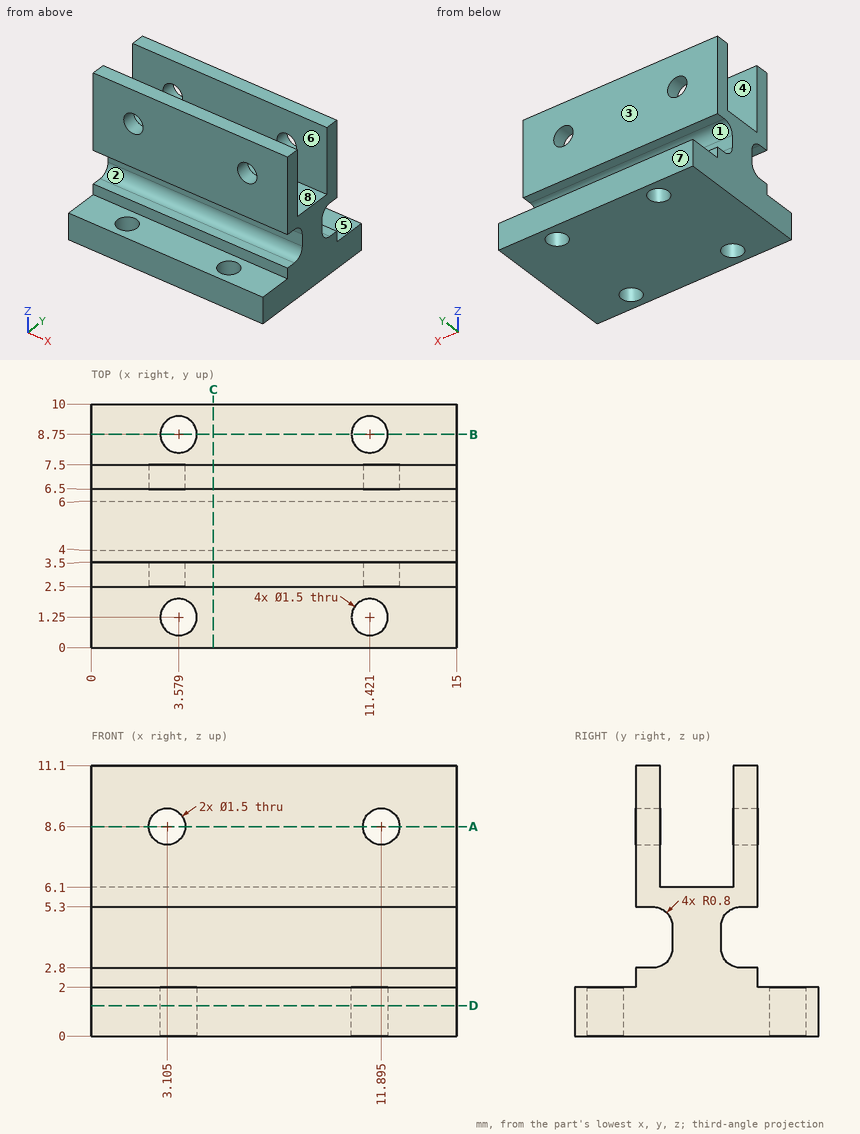
Job drawing, mm, ordinate dimensions from the low corner. One solid piece. A direction names the side the tool comes from. Round coordinates to 2 decimals unless told otherwise and drop trailing zeros. Loops run counter-clockwise (first coordinate to the right, second up) from the corner with the lowest first, then second, coordinate; pieces in that order, holes last. Notation, with made-up numbers: (86.25, 88) -> (99.25, 88) arc R30 cw to (99.25, 111) -> close; hole circle Ø7 at (51, 87). An arc over 180 degrees is marked (long way). Use a Markdown table: item, result.
1) Cut at A-A, the plane z = 8.6. List the corners of the cut face in (x, y) (1 decimal).
The answers:
| item | result |
|---|---|
| outline | (0, 2.5) -> (2.4, 2.5) -> (2.4, 3.5) -> (0, 3.5) -> close; (0, 6.5) -> (2.4, 6.5) -> (2.4, 7.5) -> (0, 7.5) -> close; (3.9, 2.5) -> (11.1, 2.5) -> (11.1, 3.5) -> (3.9, 3.5) -> close; (3.9, 6.5) -> (11.1, 6.5) -> (11.1, 7.5) -> (3.9, 7.5) -> close; (12.6, 2.5) -> (15, 2.5) -> (15, 3.5) -> (12.6, 3.5) -> close; (12.6, 6.5) -> (15, 6.5) -> (15, 7.5) -> (12.6, 7.5) -> close |
2) Pull direction Y, two halves, no side cores. Call the marked faces 5, 6, 7 and 8: pulls with the +Y half, pulls with the -Y half, needs draft (parallel to the pull), parting line crosses it, or undercut.
The answers:
| item | result |
|---|---|
| face 5 | needs draft |
| face 6 | undercut |
| face 7 | pulls with the +Y half |
| face 8 | undercut |
3) Tool access for the marked faces 1, 2, 3 and 4: list every direction of +Z, -Z, +X, -X, +Y, -Y with a clear straight run to the whole face (end or side of a thin tool).
The answers:
| item | result |
|---|---|
| face 1 | +X, -X, +Y |
| face 2 | +X, -X, -Y |
| face 3 | +Z, +X, -X, +Y |
| face 4 | +Z, +X, -X |
4) Cut at D-D, the plane z = 1.25. List the corners of the cut face in (x, y).
The answers:
| item | result |
|---|---|
| outline | (0, 0) -> (15, 0) -> (15, 10) -> (0, 10) -> close; hole circle Ø1.5 at (3.58, 1.25); hole circle Ø1.5 at (3.58, 8.75); hole circle Ø1.5 at (11.42, 1.25); hole circle Ø1.5 at (11.42, 8.75) |
5) Drop flat-ended pins along their axis: pin 1 Ø5.5 at (x, z) = (10, 7.5) entering from -Y; pin 2 Ø1.7 at (x, z) = (11.9, 8.6) entering from +Y; pin 3 Ø1 at (x, z) = (9, 4) entering from -Y; pin 4 Ø1.7 at (x, y) = (3.58, 8.75) entering from -Z. Give the stop position or say it passes through.
The answers:
| item | result |
|---|---|
| pin 1 | stops at y = 2.5 |
| pin 2 | stops at y = 7.5 |
| pin 3 | stops at y = 3.99 |
| pin 4 | stops at z = 0 |
6) Probe line 1 (Y direction, x = 9.75, z = 6.75); line 2 (Z direction, x = 3.5, y = 2.75); line 3 (X direction, y = 9, z = 1) (1 decimal). List the from-to ranges inside material, lowest first. Write a range as [from, to].
The answers:
| item | result |
|---|---|
| line 1 | y = [2.5, 3.5], [6.5, 7.5] |
| line 2 | z = [0, 2.8], [5.3, 7.96], [9.24, 11.1] |
| line 3 | x = [0, 2.9], [4.3, 10.7], [12.1, 15] |
7) Cut at C-C, the plane x = 5. List the corners of the cut face in (y, z).
The answers:
| item | result |
|---|---|
| outline | (0, 0) -> (10, 0) -> (10, 2) -> (7.5, 2) -> (7.5, 2.8) -> (6.8, 2.8) arc R0.8 cw to (6, 3.6) -> (6, 4.5) arc R0.8 cw to (6.8, 5.3) -> (7.5, 5.3) -> (7.5, 11.1) -> (6.5, 11.1) -> (6.5, 6.1) -> (3.5, 6.1) -> (3.5, 11.1) -> (2.5, 11.1) -> (2.5, 5.3) -> (3.2, 5.3) arc R0.8 cw to (4, 4.5) -> (4, 3.6) arc R0.8 cw to (3.2, 2.8) -> (2.5, 2.8) -> (2.5, 2) -> (0, 2) -> close |
8) Cut at B-B, the plane y = 8.75. List the corners of the cut face in (x, z), and give its area (3 significant figures).
The answers:
| item | result |
|---|---|
| outline | (0, 0) -> (2.83, 0) -> (2.83, 2) -> (0, 2) -> close; (4.33, 0) -> (10.67, 0) -> (10.67, 2) -> (4.33, 2) -> close; (12.17, 0) -> (15, 0) -> (15, 2) -> (12.17, 2) -> close |
| area | 24.0 mm2 |
